from build123d import *

# Parameters (mm, degrees)
SKETCH_1_R      = 2.55
SKETCH_1_W      = 15
SKETCH_1_H      = 15
SKETCH_1_W_2    = 68
SKETCH_1_H_2    = 8
EXTRUDE_1_DEPTH = 4


with BuildPart() as part:
    # 草图1 → 凸台-拉伸1 (new body)
    with BuildSketch(Plane(origin=(0, 0, 0), x_dir=(1, 0, 0), z_dir=(0, 1, 0))):
        with BuildLine():
            Line((2958.153435269, 1776.763982112), (3196.153435269, 1776.763982112))
            ThreePointArc((3196.153435269, 1776.763982112), (3200.396075956, 1775.006622799), (3202.153435269, 1770.763982112))
            Line((3202.153435269, 1770.763982112), (3202.153435269, 1662.763982112))
            ThreePointArc((3202.153435269, 1662.763982112), (3200.396075956, 1658.521341424), (3196.153435269, 1656.763982112))
            Line((3196.153435269, 1656.763982112), (2958.153435269, 1656.763982112))
            ThreePointArc((2958.153435269, 1656.763982112), (2953.910794582, 1658.521341424), (2952.153435269, 1662.763982112))
            Line((2952.153435269, 1662.763982112), (2952.153435269, 1770.763982112))
            ThreePointArc((2952.153435269, 1770.763982112), (2953.910794582, 1775.006622799), (2958.153435269, 1776.763982112))
        make_face()
        with Locations(Location((2958.153435269, 1770.763982112, 0), (0, 0, 270))):
            Circle(SKETCH_1_R, mode=Mode.SUBTRACT)
        with Locations(Location((3196.153435269, 1770.763982112, 0), (0, 0, 270))):
            Circle(SKETCH_1_R, mode=Mode.SUBTRACT)
        with Locations(Location((3077.153435269, 1766.763982112, 0), (0, 0, 270))):
            Circle(SKETCH_1_R, mode=Mode.SUBTRACT)
        with Locations(Location((2958.153435269, 1662.763982112, 0), (0, 0, 270))):
            Circle(SKETCH_1_R, mode=Mode.SUBTRACT)
        with Locations(Location((3196.153435269, 1662.763982112, 0), (0, 0, 270))):
            Circle(SKETCH_1_R, mode=Mode.SUBTRACT)
        with Locations(Location((3077.153435269, 1666.763982112, 0), (0, 0, 270))):
            Circle(SKETCH_1_R, mode=Mode.SUBTRACT)
        with Locations(Location((3196.153435269, 1716.763982112, 0), (0, 0, 270))):
            Circle(SKETCH_1_R, mode=Mode.SUBTRACT)
        with Locations(Location((2958.153435269, 1716.763982112, 0), (0, 0, 270))):
            Circle(SKETCH_1_R, mode=Mode.SUBTRACT)
        with Locations((2977.153435269, 1731.763982112)):
            Rectangle(SKETCH_1_W, SKETCH_1_H, mode=Mode.SUBTRACT)
        with Locations((3007.153435269, 1736.763982112)):
            Rectangle(SKETCH_1_W, SKETCH_1_H, mode=Mode.SUBTRACT)
        with Locations((3102.153435269, 1726.763982112)):
            Rectangle(SKETCH_1_W, SKETCH_1_H, mode=Mode.SUBTRACT)
        with Locations((3037.153435269, 1681.763982112)):
            Rectangle(SKETCH_1_W, SKETCH_1_H, mode=Mode.SUBTRACT)
        with Locations((3037.153435269, 1731.763982112)):
            Rectangle(SKETCH_1_W, SKETCH_1_H, mode=Mode.SUBTRACT)
        with Locations((3112.153435269, 1751.763982112)):
            Rectangle(SKETCH_1_W, SKETCH_1_H, mode=Mode.SUBTRACT)
        with Locations((3127.153435269, 1731.763982112)):
            Rectangle(SKETCH_1_W, SKETCH_1_H, mode=Mode.SUBTRACT)
        with Locations((3152.153435269, 1736.763982112)):
            Rectangle(SKETCH_1_W, SKETCH_1_H, mode=Mode.SUBTRACT)
        with Locations((3127.153435269, 1706.763982112)):
            Rectangle(SKETCH_1_W, SKETCH_1_H, mode=Mode.SUBTRACT)
        with Locations((3177.153435269, 1706.763982112)):
            Rectangle(SKETCH_1_W, SKETCH_1_H, mode=Mode.SUBTRACT)
        with Locations((3152.153435269, 1711.763982112)):
            Rectangle(SKETCH_1_W, SKETCH_1_H, mode=Mode.SUBTRACT)
        with Locations((3102.153435269, 1701.763982112)):
            Rectangle(SKETCH_1_W, SKETCH_1_H, mode=Mode.SUBTRACT)
        with Locations((3117.153435269, 1681.763982112)):
            Rectangle(SKETCH_1_W, SKETCH_1_H, mode=Mode.SUBTRACT)
        with Locations((3177.153435269, 1731.763982112)):
            Rectangle(SKETCH_1_W, SKETCH_1_H, mode=Mode.SUBTRACT)
        with Locations((3007.153435269, 1761.763982112)):
            Rectangle(SKETCH_1_W_2, SKETCH_1_H_2, mode=Mode.SUBTRACT)
    extrude(amount=EXTRUDE_1_DEPTH)


solid = part.part
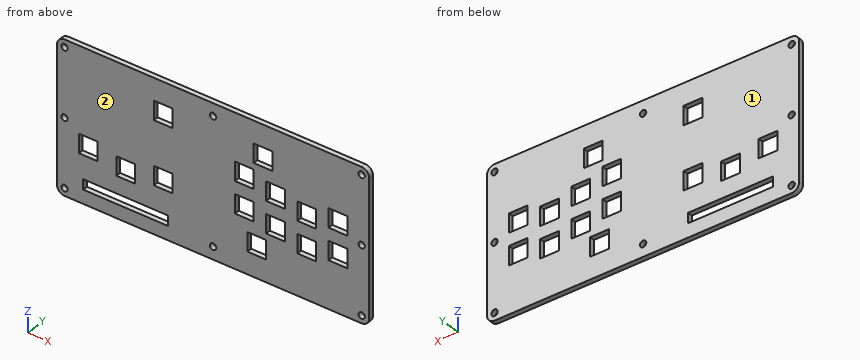
CAD build for the part. Positions are in the model's coordinates, mm. Face numbers are marked on the shaded views. Coordinates: 2 decimals unless noted, no trailing zeros. Write each loop counter-clockwise with the first axis right and the second up, starting at its lowest first coordinate (ties: lowest second). Pieces come first, ordered by that corner, then holes. Notation, with made-up numbers: M 24,56.25 L 36,56.25 A31 ccw 36,88.25 Z; hole C -10.5,54.25 d3. An arc over 180 degrees is marked long. Answer as a JSON object with one key per item and string values. Group by question number.
1) Saw through at C-C (x = 3036). Write the cut outline in (y, z), plus the area to 3 significant figures.
2) Saw through at B-B (x = 3147.5). Write the cut outline in (y, z).
3) Saw through at A-A (z = -1737). Write the cut outline in (x, y), plus the area to 3 significant figures.
4) Saw through at D-D (z = -1682). Write the cut outline in (x, y).
5) Wall check: line 1 (Z direction, x = 3132.5, y = 2.6); line 2 (X direction, y = 0.65, z = -1711); line 3 (Z direction, x = 3032, y = 1.6). Give the ranges that are in metal, low to high. Write a range as from..to.
6) Mould opens along Y. For the marked faces 1 and 2 say: +Y half, -Y half, draft (parallel to the pull), parting line (faces both ways), or undercut.
Values follow:
{
 "1": {"outline": "M 0,-1776.76 L 4,-1776.76 L 4,-1765.76 L 0,-1765.76 Z; M 0,-1757.76 L 4,-1757.76 L 4,-1739.26 L 0,-1739.26 Z; M 0,-1724.26 L 4,-1724.26 L 4,-1689.26 L 0,-1689.26 Z; M 0,-1674.26 L 4,-1674.26 L 4,-1656.76 L 0,-1656.76 Z", "area": "328 mm2"},
 "2": {"outline": "M 0,-1776.76 L 4,-1776.76 L 4,-1744.26 L 0,-1744.26 Z; M 0,-1729.26 L 4,-1729.26 L 4,-1719.26 L 0,-1719.26 Z; M 0,-1704.26 L 4,-1704.26 L 4,-1656.76 L 0,-1656.76 Z"},
 "3": {"outline": "M 2952.15,0 L 2969.65,0 L 2969.65,4 L 2952.15,4 Z; M 2984.65,0 L 2999.65,0 L 2999.65,4 L 2984.65,4 Z; M 3014.65,0 L 3029.65,0 L 3029.65,4 L 3014.65,4 Z; M 3044.65,0 L 3119.65,0 L 3119.65,4 L 3044.65,4 Z; M 3134.65,0 L 3144.65,0 L 3144.65,4 L 3134.65,4 Z; M 3159.65,0 L 3169.65,0 L 3169.65,4 L 3159.65,4 Z; M 3184.65,0 L 3202.15,0 L 3202.15,4 L 3184.65,4 Z", "area": "640 mm2"},
 "4": {"outline": "M 2952.15,0 L 3029.65,0 L 3029.65,4 L 2952.15,4 Z; M 3044.65,0 L 3109.65,0 L 3109.65,4 L 3044.65,4 Z; M 3124.65,0 L 3202.15,0 L 3202.15,4 L 3124.65,4 Z"},
 "5": {"line 1": "z = -1776.76..-1739.26, -1724.26..-1714.26, -1699.26..-1656.76", "line 2": "x = 2952.15..3119.65, 3134.65..3144.65, 3159.65..3169.65, 3184.65..3202.15", "line 3": "z = -1776.76..-1765.76, -1757.76..-1739.26, -1724.26..-1689.26, -1674.26..-1656.76"},
 "6": {"face 1": "+Y half", "face 2": "-Y half"}
}
